Source: CAD feature listing. Evaluate the final solid. Frame: model axes, mm. A direction names the side the tool comes from. Coordinates: 2 decimals unless noted, no trailing zeros. Order: outer loops, then holes, each group sorted by start corner. A loop starts at its lowest first (then second) coordinate and runs counter-clockwise, first axis right, second up. Notation, with made-up numbers: (33, 28) -> (78, 28) arc R17 ccw to (78, 45) -> close; hole circle Ø6 at (-35, -4.5). An arc over 180 degrees is marked (long way). Write item = value, one per line. Start each with the question number.
Item 1: Section query D-D (x = 10). Output: boundary loops of the cut face in (y, z), then the cut area to 3 significant figures.
Item 2: Section query C-C (z = 5). Output: boundary loops of the cut face in (x, y).
Item 3: Set-up query: faces 5 (the cylindrical face through (46.93, 18.5, -21.54)), 6 (the flat face through (0, 19, -13)). Return all of +Z, -Z, +X, -X, +Y, -Y with unobstructed straight access to the full face (end or side cutting, diameter ignored); none if empty.
Item 4: Section query B-B (y = 4). Output: boundary loops of the cut face in (x, z).
Item 5: Section query A-A (x = 19.05). Output: boundary loops of the cut face in (y, z), then the cut area to 3 significant figures.
Item 6: Ray query, line 1 along X through (y, z) = (19.05, -19.75); line 2 along Y through (x, z) = (44.45, -22.5); line 3 along Z through (x, y) = (41.5, 24.5). Return the intervals inside material, ascending. Write a range as [from, to].
Item 7: Mould query, pull axis X, two halves, no side actions, for faces 1 (the flat face through (63.5, 19, -13)), 2 (the cylindrical face through (24.916, 21.482, 12.522)), 3 (the flat face through (31, 19, 0)), 4 (the conical face through (44.89, 18.99, -16.52)). Classes: released by +X, released by -X, zero draft, split by the parting line, or undercut.
Item 8: Contact query for flat-ended pins moving along their axis: pin 1 (8 mm diameter, centred on x = 44.45, y = 19.05, fed in from +Z); pin 2 (1.5 mm diameter, centred on y = 22, z = 14, fed in from -X). Output: stop coordinate, or through.
Autodesk Inventor part; units mm, degrees
ref_plane "YZ Plane" through (0, 0, 0) normal (1, 0, 0) x (0, 1, 0)
ref_plane "XZ Plane" through (0, 0, 0) normal (0, 1, 0) x (-1, 0, 0)
ref_plane "XY Plane" through (0, 0, 0) normal (0, 0, 1) x (1, 0, 0)
sketch "Sketch1" plane through (0, 0, 0) normal (0, 0, 1) x (1, 0, 0)
  line L0 (0, 0) -> (63.5, 0)
  line L1 (63.5, 0) -> (63.5, 38.1)
  line L2 (63.5, 38.1) -> (0, 38.1)
  line L3 (0, 38.1) -> (0, 0)
  circle A0 centre (19.05, 19.05) radius 6.35
  dimension "d0" = 63.5
  dimension "d1" = 38.1
  dimension "d4" = 19.05
  dimension "d5" = 12.7
extrude "Extrusion1" add sketch "Sketch1" against normal blind 25.4 contours L3 L2 L1 L0 | A0
extrude "Extrusion2" add sketch "Sketch1" along normal blind 25.4 contours A0
sketch "Sketch2" plane through (0, 0, -25.4) normal (0, 0, -1) x (-1, 0, 0)
  line L0 (-63.5, 0) -> (-63.5, 38.1)
  circle A0 centre (-44.45, 19.05) radius 8.4036
  dimension "d8" = 19.05
hole "Hole1" at (44.45, 19.05, -25.4) direction (0, 0, 1) diameter 5.08 depth 7.62 tip angle 118
properties part number "proxycimulator775"
Computed:
q1.outline = (0, -25.4) -> (38.1, -25.4) -> (38.1, 0) -> (0, 0) -> close
q1.area = 968 mm^2
q2.outline = circle Ø12.7 at (19.05, 19.05)
q3.face_5 = -Z
q3.face_6 = +Z, -Z, -X, +Y, -Y
q4.outline = (0, -25.4) -> (63.5, -25.4) -> (63.5, 0) -> (0, 0) -> close
q5.outline = (0, -25.4) -> (38.1, -25.4) -> (38.1, 0) -> (25.4, 0) -> (25.4, 25.4) -> (12.7, 25.4) -> (12.7, 0) -> (0, 0) -> close
q5.area = 1,290 mm^2
q6.line_1 = [0, 41.91], [46.99, 63.5]
q6.line_2 = [0, 16.51], [21.59, 38.1]
q6.line_3 = [-25.4, 0]
q7.face_1 = released by +X
q7.face_2 = split by the parting line
q7.face_3 = zero draft
q7.face_4 = undercut
q8.pin_1 = 0
q8.pin_2 = 13.09
